Input: part model. Units: mm. Frame: model coordinates. Face numbers are marked on the shaded views. A direction names the side the tool comes from. Round coordinates to 2 decimals unless told otherwise and drop trailing zeros. Write each loop counter-clockwise with the first axis right and the second up, starting at its lowest first coordinate (ties: lowest second). Pieces come first, ordered by that corner, then holes. Notation, with made-up numbers: (42.25, -9.75) -> (58.25, -9.75) arc R19 cw to (58.25, 17.25) -> close; hole circle Ø2 at (-28, -31). An arc over 180 degrees is marked (long way). Write item = value, one per line.
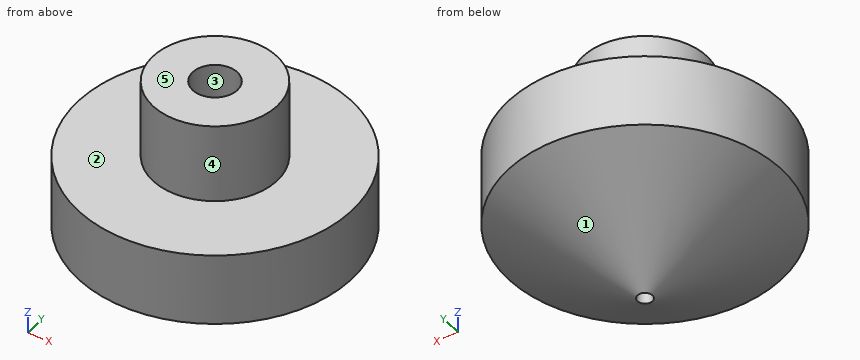
```python
from build123d import *

# Parameters (mm, degrees)
F2_R     = 4.7625
F4_DEPTH = 25.4
F5_R     = 1.5875
F6_DEPTH = 25.4


with BuildPart() as f1:
    # F0 (on Front) → F1 (revolve)
    with BuildSketch(Plane.XZ):
        Polygon((0, 49.591192), (0, 0), (29.094543, 17.542299), (29.094543, 32.854902), (13.208, 32.854902), (13.208, 49.591192), align=None)
    revolve(axis=Axis((0, 0, 24.795596), (0, 0, 1)))

    # F2 (on face) → F4 (cut)
    with BuildSketch(Plane.XY.offset(49.591192)):
        Circle(F2_R)
    extrude(amount=-F4_DEPTH, mode=Mode.SUBTRACT)

    # F5 (on Top) → F6 (cut)
    with BuildSketch(Plane.XY):
        Circle(F5_R)
    extrude(amount=F6_DEPTH, mode=Mode.SUBTRACT)


solid = f1.part
```
1) Cut plane D-D (z = 45.5). Return the cut outline in (x, y) (1 decimal).
Solutions:
outline = circle Ø26.4 at (0, 0); hole circle Ø9.5 at (0, 0)
2) First-contact query: P1, Ø8, axis at y = 3.5, z = 38, coming from the -X side; P2, Ø10, axis at y = -12.5, z = 34.5, coming from the -X side; P3, Ø3, axis at y = -4.5, z = 41, coming from the +X side. Flat tips, straight axial feed; report the tip coordinate or a pass-through.
Solutions:
P1 = -13.21
P2 = -28.04
P3 = 12.86
3) Cut plane A-A (x = 0). Return the cut outline in (y, z), and give its area (3 significant figures).
Solutions:
outline = (-29.09, 17.54) -> (-1.59, 0.96) -> (-1.59, 24.19) -> (-4.76, 24.19) -> (-4.76, 49.59) -> (-13.21, 49.59) -> (-13.21, 32.85) -> (-29.09, 32.85) -> close; (1.59, 0.96) -> (29.09, 17.54) -> (29.09, 32.85) -> (13.21, 32.85) -> (13.21, 49.59) -> (4.76, 49.59) -> (4.76, 24.19) -> (1.59, 24.19) -> close
area = 1,530 mm^2
4) Line query: L1, parallel to Y at x = 0, z = 7.25; L2, parallel to X at y = 0, z = 16.75; L3, parallel to Y at x = 0, z = 11. Output: solid intervals per line, ascending. Write a range as from..to.
Solutions:
L1 = -12.02..-1.59, 1.59..12.02
L2 = -27.78..-1.59, 1.59..27.78
L3 = -18.24..-1.59, 1.59..18.24
5) Draft query along Y for the marked faces 1, 2 and 3. Return one class per face: +Y half, -Y half, draft (parallel to the pull), parting line (faces both ways), or undercut.
Solutions:
face_1 = parting line
face_2 = draft
face_3 = undercut
6) Cut plane C-C (z = 22.5). Return the cut outline in (x, y) (1 decimal), and give its area (3 significant figures).
Solutions:
outline = circle Ø58.2 at (0, 0); hole circle Ø3.2 at (0, 0)
area = 2,650 mm^2
7) Access query for the marked faces 4 and 5. Directions: +Z, -Z, +X, -X, +Y, -Y. A direction counts if a zero-diameter tool reaches every point of the face in a straight line with its end or side. Return the directions, or none.
Solutions:
face_4 = +Z
face_5 = +Z, +X, -X, +Y, -Y
